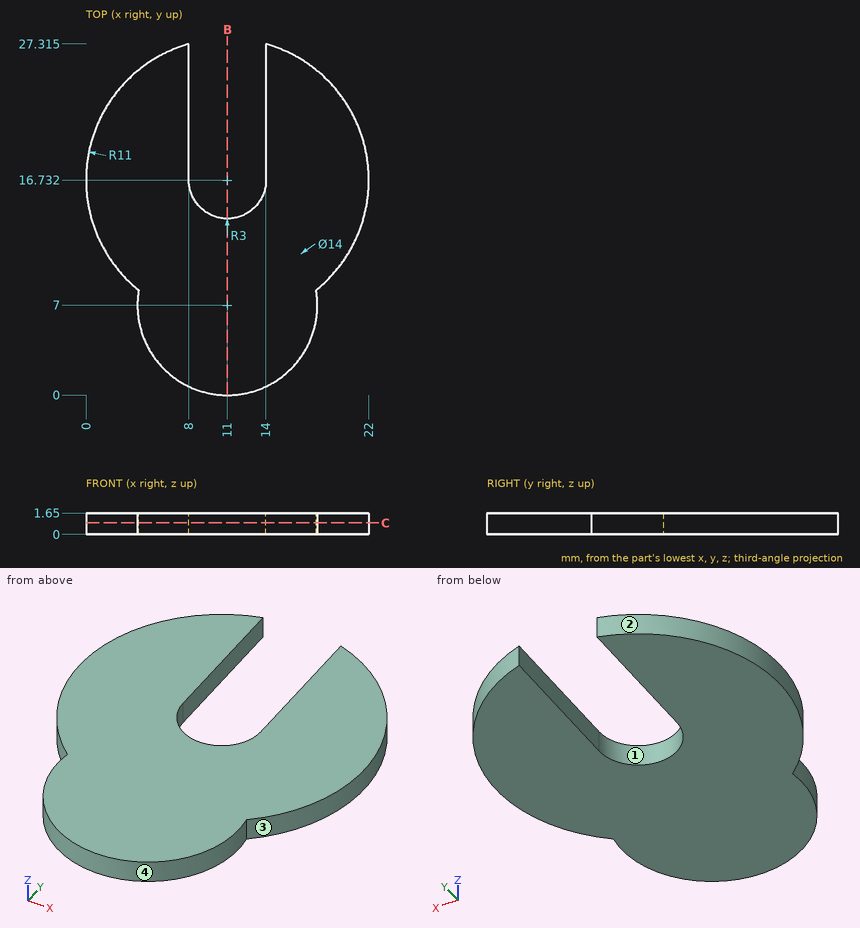
Source: three-view drawing plus pictorial views. Frame: mm from the lowest corner of the part. Give positions to 0.01 mm unless a question says otherwise; leave off trailing zeros. Order: outer loops, then holes, each group sorted by start corner. A loop starts at its lowest first (then second) coordinate and runs counter-clockwise, first axis right, second up. Notation, with made-up numbers: (87, -39.5) - (112, -39.5) arc R16 cw to (112, -19.5) - close; hole circle Ø1 at (42.5, 52.25). An arc over 180 degrees is marked (long way). Put each result on its own line as item: value.
Item 1: Section query B-B, the plane x = 11. Return loops of the section in (y, z).
Found:
outline: (0, 0) - (13.73, 0) - (13.73, 1.65) - (0, 1.65) - close
Item 2: Draft query along X for the marked faces 1, 2, 3 and 4. Return one class per face: +X half, -X half, draft (parallel to the pull), parting line (faces both ways), or undercut.
Found:
face 1: undercut
face 2: -X half
face 3: +X half
face 4: parting line
Item 3: Ray query, L1, parallel to X at y = 23.5, z = 0.1; L2, parallel to X at y = 14.25, z = 1.1 (1 decimal); L3, parallel to X at y = 12.75, z = 1.3 (1 decimal). Return the intervals inside material, ascending. Write a range as from..to.
Found:
L1: x = 2.33..8, 14..19.67
L2: x = 0.3..9.3, 12.7..21.7
L3: x = 0.7..21.3
Item 4: Section query C-C, the plane z = 0.9. Return loops of the section in (x, y) (1 decimal), then the cut area to 3 significant figures.
Found:
outline: (4.1, 8.2) arc R7 ccw (long way) to (17.9, 8.2) arc R11 ccw to (14, 27.3) - (14, 16.7) arc R3 cw to (8, 16.7) - (8, 27.3) arc R11 ccw to start
area: 371 mm^2
